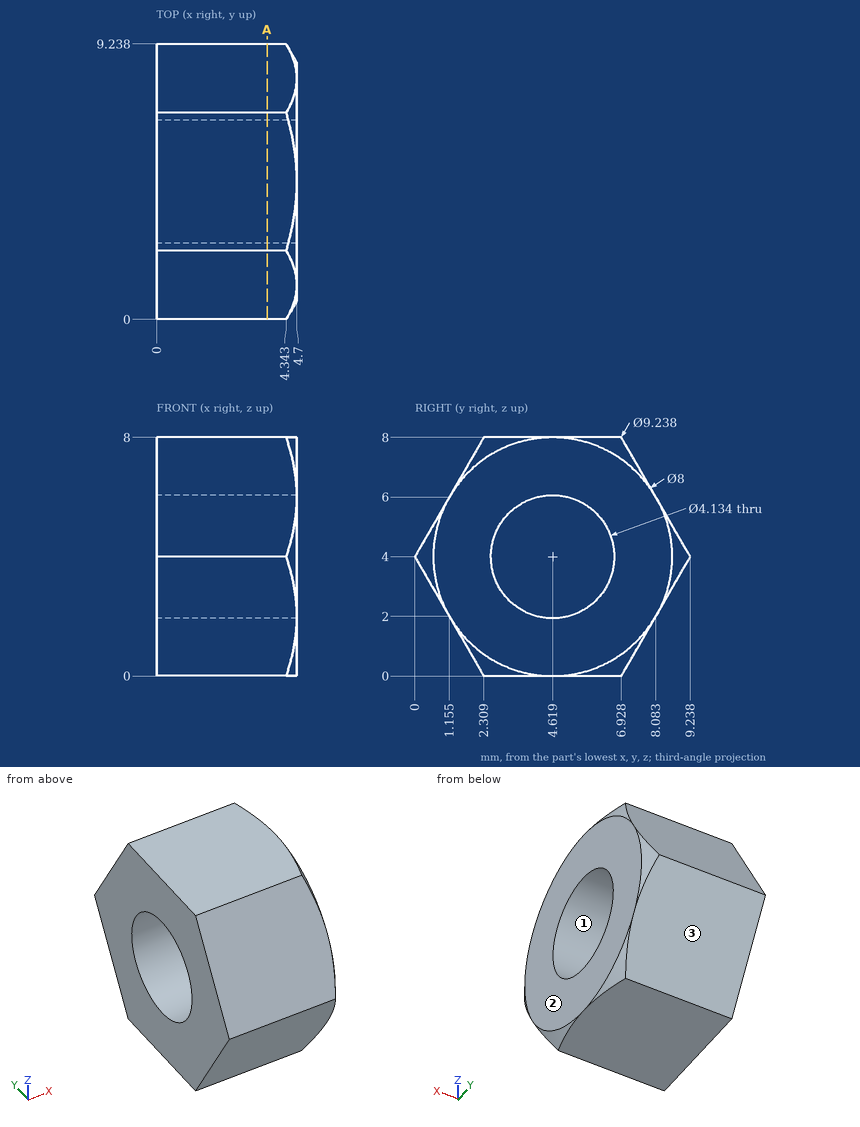
The figure shows three views and two pictorial views of one solid part (mm, origin at its lowest corner). Answer the questions. Give positions to 0.01 mm unless a question says otherwise; leave off trailing zeros. Loops run counter-clockwise (first coordinate to the right, second up) from the corner with the lowest first, then second, coordinate; pieces in that order, holes last. Notation, with made-up numbers: (39.25, -33.75) -> (62.25, -33.75) arc R30 cw to (62.25, 4.25) -> close; hole circle Ø9 at (23, -9). An arc over 180 degrees is marked (long way). Use CSV: the item, a comma, the result in double quotes.
1. Straight lines are drawn through the part: line 1 (Z direction, x = 2.4, y = 4.5); line 2 (Z direction, x = 2.05, y = 3) (1 decimal); line 3 (Y direction, x = 2.85, z = 4.25) (1 decimal). For each, find the intervals that lie inside material, in ascending order.
Found:
line 1,"0 to 1.94, 6.06 to 8"
line 2,"0 to 2.7, 5.3 to 8"
line 3,"0.1 to 2.6, 6.7 to 9.1"
2. The mould has two halves that part along Y. Classify the marked faces 1, 2 and 3: +Y half, -Y half, draft (parallel to the pull), parting line (faces both ways), or undercut.
Found:
face 1,"undercut"
face 2,"draft"
face 3,"+Y half"
3. Flat-ended cylindrical pins translate along their axes: pin 1 Ø2 at (x, z) = (1.5, 1) entering from -Y (1 decimal); pin 2 Ø3.5 at (y, z) = (4.62, 4) entering from +X. Find the tip coordinate at first contact, or state that the pin passes through.
Found:
pin 1,"y = 1.2"
pin 2,"through"
4. The part is cut by section A-A (x = 3.7). Write down the section's boundary in (y, z), then the cut area to 3 significant figures.
Found:
outline,"(0, 4) -> (2.31, 0) -> (6.93, 0) -> (9.24, 4) -> (6.93, 8) -> (2.31, 8) -> close; hole circle Ø4.13 at (4.62, 4)"
area,"42.0 mm^2"
